Source: CAD feature listing. Evaluate the final solid. Frame: model axes, mm. A direction names the side the tool comes from. Give positions to 0.01 mm unless a question says otherwise; leave off trailing zeros. Loops run counter-clockwise (first coordinate to the right, second up) from the corner with the lowest first, then second, coordinate; pieces in that order, holes last. Notation, with made-up numbers: M 29,24 L 45,24 A19 cw 45,31 Z; hole C 9,3.25 d9. An arc over 180 degrees is marked long. Answer in a Markdown table with one row per item.
```python
from build123d import *

# Parameters (mm, degrees)
SKETCH1_R           = 20
BOSS_EXTRUDE1_DEPTH = 14


with BuildPart() as part:
    # Sketch1 → Boss-Extrude1 (new, symmetric)
    with BuildSketch(Plane.XY):
        with BuildLine():
            Line((58.887604808, 11.5), (81.791697995, 11.5))
            ThreePointArc((81.791697995, 11.5), (139.5, 0), (81.791697995, -11.5))
            Line((81.791697995, -11.5), (58.887604808, -11.5))
            ThreePointArc((58.887604808, -11.5), (51.961524227, -30), (39.403094547, -45.248161732))
            Line((39.403094547, -45.248161732), (50.855141141, -65.083688282))
            ThreePointArc((50.855141141, -65.083688282), (69.75, -120.810543828), (30.936556854, -76.583688282))
            Line((30.936556854, -76.583688282), (19.48451026, -56.748161732))
            ThreePointArc((19.48451026, -56.748161732), (0, -60), (-19.48451026, -56.748161732))
            Line((-19.48451026, -56.748161732), (-30.936556854, -76.583688282))
            ThreePointArc((-30.936556854, -76.583688282), (-69.75, -120.810543828), (-50.855141141, -65.083688282))
            Line((-50.855141141, -65.083688282), (-39.403094547, -45.248161732))
            ThreePointArc((-39.403094547, -45.248161732), (-51.961524227, -30), (-58.887604808, -11.5))
            Line((-58.887604808, -11.5), (-81.791697995, -11.5))
            ThreePointArc((-81.791697995, -11.5), (-139.5, 0), (-81.791697995, 11.5))
            Line((-81.791697995, 11.5), (-58.887604808, 11.5))
            ThreePointArc((-58.887604808, 11.5), (-51.961524227, 30), (-39.403094547, 45.248161732))
            Line((-39.403094547, 45.248161732), (-50.855141141, 65.083688282))
            ThreePointArc((-50.855141141, 65.083688282), (-69.75, 120.810543828), (-30.936556854, 76.583688282))
            Line((-30.936556854, 76.583688282), (-19.48451026, 56.748161732))
            ThreePointArc((-19.48451026, 56.748161732), (0, 60), (19.48451026, 56.748161732))
            Line((19.48451026, 56.748161732), (30.936556854, 76.583688282))
            ThreePointArc((30.936556854, 76.583688282), (69.75, 120.810543828), (50.855141141, 65.083688282))
            Line((50.855141141, 65.083688282), (39.403094547, 45.248161732))
            ThreePointArc((39.403094547, 45.248161732), (51.961524227, 30), (58.887604808, 11.5))
        make_face()
        with Locations((109.5, 0)):
            Circle(SKETCH1_R, mode=Mode.SUBTRACT)
        with Locations((54.75, -94.829781714)):
            Circle(SKETCH1_R, mode=Mode.SUBTRACT)
        with Locations((-54.75, -94.829781714)):
            Circle(SKETCH1_R, mode=Mode.SUBTRACT)
        with Locations((-109.5, 0)):
            Circle(SKETCH1_R, mode=Mode.SUBTRACT)
        with Locations((-54.75, 94.829781714)):
            Circle(SKETCH1_R, mode=Mode.SUBTRACT)
        with Locations((54.75, 94.829781714)):
            Circle(SKETCH1_R, mode=Mode.SUBTRACT)
        with BuildLine():
            Line((-25.529394822, 11.5), (-35, 11.5))
            Line((-35, 11.5), (-35, -11.5))
            Line((-35, -11.5), (-25.529394822, -11.5))
            ThreePointArc((-25.529394822, -11.5), (0, -28), (25.529394822, -11.5))
            Line((25.529394822, -11.5), (35, -11.5))
            Line((35, -11.5), (35, 11.5))
            Line((35, 11.5), (25.529394822, 11.5))
            ThreePointArc((25.529394822, 11.5), (0, 28), (-25.529394822, 11.5))
        make_face(mode=Mode.SUBTRACT)
    extrude(amount=BOSS_EXTRUDE1_DEPTH, both=True)


solid = part.part
```
Q1. Section query A-A (x = -109.5). Output: boundary loops of the cut face in (y, z).
Values follow:
| item | result |
|---|---|
| outline | M -30,-14 L -20,-14 L -20,14 L -30,14 Z; M 20,-14 L 30,-14 L 30,14 L 20,14 Z |
Q2. Section query D-D (y = -100.5). Output: boundary loops of the cut face in (x, z), plus the area to 3 significant figures.
Values follow:
| item | result |
|---|---|
| outline | M -84.21,-14 L -73.93,-14 L -73.93,14 L -84.21,14 Z; M -35.57,-14 L -25.29,-14 L -25.29,14 L -35.57,14 Z; M 25.29,-14 L 35.57,-14 L 35.57,14 L 25.29,14 Z; M 73.93,-14 L 84.21,-14 L 84.21,14 L 73.93,14 Z |
| area | 1,150 mm^2 |
Q3. Contact query for flat-ended pins moving along their axis: pin 1 Ø1.5 at (y, z) = (-69, 9.5) entering from +X; pin 2 Ø1 at (x, z) = (74.5, 9.5) entering from +Y; pin 3 Ø10.5 at (x, z) = (29.5, -5.5) entering from -Y; pin 4 Ø11.5 at (y, z) = (-3, 3.5) entering from -X. Output: stop coordinate, or through.
Values follow:
| item | result |
|---|---|
| pin 1 | x = 71.21 |
| pin 2 | y = 117.84 |
| pin 3 | y = -117.19 |
| pin 4 | x = -139.5 |
Q4. Ray query, probe 1 along X at (y, z) = (95.5, 11.75); probe 2 along X at (y, z) = (-24.5, 9); probe 3 along Y at (x, z) = (-47.5, -8.25). Return the intervals inside material, ascending. Write a range as from..to.
Values follow:
| item | result |
|---|---|
| probe 1 | -84.74..-74.74, -34.76..-24.76, 24.76..34.76, 74.74..84.74 |
| probe 2 | -126.81..-92.19, -54.77..-13.56, 13.56..54.77, 92.19..126.81 |
| probe 3 | -123.94..-113.47, -76.19..-59.27, -36.66..36.66, 59.27..76.19, 113.47..123.94 |
Q5. Mould query, pull axis X, two halves, no side actions, for faces 1 (the cylindrical face through (52.1, -29.76, 0.2)), 2 (the flat face through (-20, 28, 14)). Classes: +X half, -X half, draft (parallel to the pull), parting line (faces both ways), or undercut.
Values follow:
| item | result |
|---|---|
| face 1 | undercut |
| face 2 | draft |
Q6. Section query B-B (y = 0). Output: boundary loops of the cut face in (x, z).
Values follow:
| item | result |
|---|---|
| outline | M -139.5,-14 L -129.5,-14 L -129.5,14 L -139.5,14 Z; M -89.5,-14 L -35,-14 L -35,14 L -89.5,14 Z; M 35,-14 L 89.5,-14 L 89.5,14 L 35,14 Z; M 129.5,-14 L 139.5,-14 L 139.5,14 L 129.5,14 Z |
Q7. Section query C-C (x = 45.5). Output: boundary loops of the cut face in (y, z).
Values follow:
| item | result |
|---|---|
| outline | M -123.37,-14 L -112.56,-14 L -112.56,14 L -123.37,14 Z; M -77.1,-14 L -55.81,-14 L -55.81,14 L -77.1,14 Z; M -39.11,-14 L 39.11,-14 L 39.11,14 L -39.11,14 Z; M 55.81,-14 L 77.1,-14 L 77.1,14 L 55.81,14 Z; M 112.56,-14 L 123.37,-14 L 123.37,14 L 112.56,14 Z |
Q8. Reachability of faces 3 (the flat face through (-20, 28, -14)), 4 (the flat face through (30, 11.5, 0)) from +Z, -Z, +X, -X, +Y, -Y: full face, straight path, thin tool, end or side. Return the list, or none.
Values follow:
| item | result |
|---|---|
| face 3 | -Z, +X, -X, +Y, -Y |
| face 4 | +Z, -Z |
